Input: part model. Units: mm. Frame: model coordinates. Coordinates: 2 decimals unless noted, no trailing zeros. Loops run counter-clockwise (first coordinate to the right, second up) from the corner with the lowest first, then second, coordinate; pieces in that order, holes last.
(1) Line query: L1, parallel to X at y = 2.75, z = 0; L2, parallel to X at y = 3, z = -1.25; L3, parallel to Z at x = 43.5, y = 5. Output: solid intervals per line, ascending.
(2) Section A-A, the plane x = 0. Return loops of the section in (y, z).
(3) Section D-D, the plane x = -45.5. Return loops of the section in (y, z), then the cut area to 3 significant figures.
(4) Section C-C, the plane y = 3.25. Return loops of the section in (x, z).
(5) Contact query for flat-ended pins moving along their axis: P1, Ø3, axis at x = -15, y = 3.5, coming from the +Z side; P2, Ø3, axis at x = -46, y = 4.5, coming from the -Z side; P3, Ø4, axis at x = 0, z = 0, coming from the -Y side. Output: stop coordinate, or through.
(6) Section B-B, the plane z = 0. Return loops of the section in (x, y), then the cut area to 3 significant figures.
```python
from build123d import *

# Parameters (mm, degrees)
SKETCH1_R           = 6.5
SKETCH1_R_2         = 2.5
BOSS_EXTRUDE1_DEPTH = 7
BOSS_EXTRUDE2_START = 4
BOSS_EXTRUDE2_DEPTH = 56
CIRPATTERN1_COUNT   = 2


with BuildPart() as part:
    # Sketch1 → Boss-Extrude1 (new body)
    with BuildSketch(Plane(origin=(0, 0, 0), x_dir=(1, 0, 0), z_dir=(0, 1, 0))):
        with Locations(Location((0, 0, 0), (0, 0, 270))):
            Circle(SKETCH1_R)
        with Locations(Location((0, 0, 0), (0, 0, 270))):
            Circle(SKETCH1_R_2, mode=Mode.SUBTRACT)
    extrude(amount=BOSS_EXTRUDE1_DEPTH)

    # Sketch2 → Boss-Extrude2 (add)
    with BuildSketch(Plane(origin=(0, 0, 0), x_dir=(0, 0, -1), z_dir=(1, 0, 0)).offset(BOSS_EXTRUDE2_START)):
        with BuildLine():
            ThreePointArc((-4.4023555, 5.870499115), (0.805969699, 4.99680087), (4.4023555, 1.129500885))
            Line((4.4023555, 1.129500885), (-4.4023555, 5.870499115))
        make_face()
        with BuildLine():
            Line((-4.4023555, 5.870499115), (4.4023555, 1.129500885))
            ThreePointArc((4.4023555, 1.129500885), (-0.805969699, 2.00319913), (-4.4023555, 5.870499115))
        make_face()
    boss_extrude2 = extrude(amount=BOSS_EXTRUDE2_DEPTH)

    # CirPattern1: Boss-Extrude2 ×2 about axis
    cirpattern1_axis = Axis((0, 7.76683161, 0), (0, -1, 0))
    for i in range(1, CIRPATTERN1_COUNT):
        add(boss_extrude2.rotate(cirpattern1_axis, i * 360 / CIRPATTERN1_COUNT))


solid = part.part
```
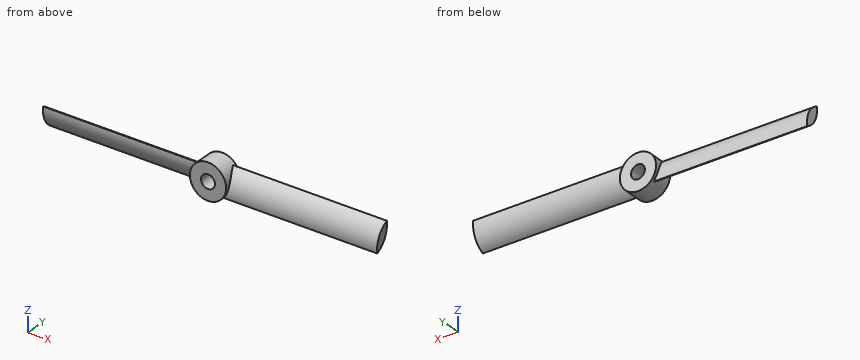
Report:
1. L1: x = -60 to -2.5, 2.5 to 60
1. L2: x = -60 to -2.17, 2.17 to 60
1. L3: z = -0.8 to 3.95
2. outline: (0, -6.5) - (7, -6.5) - (7, -2.5) - (0, -2.5) - close; (0, 2.5) - (7, 2.5) - (7, 6.5) - (0, 6.5) - close
3. outline: (1.13, 4.4) arc R8.2 ccw to (5.87, -4.4) arc R8.2 ccw to start
3. area: 23.2 mm2
4. outline: (-60, -2.54) - (-5.98, -2.54) arc R6.5 ccw to (5.75, -3.02) - (60, -3.02) - (60, 2.54) - (5.98, 2.54) arc R6.5 ccw to (-5.75, 3.02) - (-60, 3.02) - close; hole circle Ø5 at (0, 0)
5. P1: stops at z = 3.95
5. P2: stops at z = -4.4
5. P3: passes through
6. outline: (-60, 1.62) - (-6.5, 1.62) - (-6.5, 0) - (-2.5, 0) - (-2.5, 7) - (-6.5, 7) - (-6.5, 5.38) - (-60, 5.38) - close; (2.5, 0) - (6.5, 0) - (6.5, 1.62) - (60, 1.62) - (60, 5.38) - (6.5, 5.38) - (6.5, 7) - (2.5, 7) - close
6. area: 457 mm2
